```python
from build123d import *

# Parameters (mm, degrees)
SKETCH1_W           = 30
SKETCH1_H           = 9
BOSS_EXTRUDE1_DEPTH = 4
SKETCH2_W           = 34
SKETCH2_H           = 13
SKETCH2_W_2         = 30
SKETCH2_H_2         = 9
BOSS_EXTRUDE2_DEPTH = 36


with BuildPart() as part:
    # Sketch1 → Boss-Extrude1 (new body)
    with BuildSketch(Plane.XY):
        Polygon((-17, 6.5), (-17, -6.5), (-5.5, -6.5), (-5.5, -5.5), (5.5, -5.5), (5.5, -6.5), (17, -6.5), (17, 6.5), align=None)
        Rectangle(SKETCH1_W, SKETCH1_H, mode=Mode.SUBTRACT)
    extrude(amount=BOSS_EXTRUDE1_DEPTH)

    # Sketch2 → Boss-Extrude2 (add)
    with BuildSketch(Plane.XY.offset(4)):
        Rectangle(SKETCH2_W, SKETCH2_H)
        Rectangle(SKETCH2_W_2, SKETCH2_H_2, mode=Mode.SUBTRACT)
    extrude(amount=BOSS_EXTRUDE2_DEPTH)


solid = part.part
```
Model file for the job. Use its own axes, mm. A direction names the side the tool comes from. Give positions to 0.01 mm unless a question says otherwise; leave off trailing zeros. Write each loop counter-clockwise with the first axis right and the second up, starting at its lowest first coordinate (ties: lowest second). Pieces come first, ordered by that corner, then holes. Notation, with made-up numbers: (-11, 76.5) -> (17, 76.5) arc R18 cw to (17, 98.5) -> close; hole circle Ø11 at (28, 8.25). An arc over 180 degrees is marked (long way). Use CSV: the item, a comma, the result in double quotes. Start each with the question number.
1) Cut at A-A on x = -10. List the corners of the cut face in (y, z), plus the area to 3 significant figures.
2) Pin check, flat tips, straight feed: P1, Ø2, axis at x = -11, y = -2, coming from the +Z side; P2, Ø0.8, axis at x = -1.5, y = -6, coming from the -Z side; P3, Ø2, axis at x = 2.5, z = 2, coming from the -Y side. Stop position of each tip, or through.
3) Drill centre lines: L1, parallel to Y at x = 1.5, z = 16; L2, parallel to X at y = -1, z = 24. Where is each one in solid material? Low to high.
4) Two-plate mould, pull along Y, no slides. Class faces 1 (the flat face through (0, 6.5, 20)), 2 (the flat face through (0, -5.5, 2)), 3 (the flat face through (5.5, -6, 2)), 4 (the flat face through (0, 4.5, 20)): released by +Y, released by -Y, zero draft, split by the parting line, or undercut.
5) Tool access for faces 5 (the flat face through (0, -4.5, 20)), 6 (the flat face through (17, 0, 20)), 7 (the flat face through (-5.5, -6, 2)): list every direction of +Z, -Z, +X, -X, +Y, -Y with a clear straight run to the whole face (end or side of a thin tool).
6) Cut at B-B on z = 31. List the corners of the cut face in (x, y), plus the area to 3 significant figures.
7) Cut at C-C on y = -2.25. List the corners of the cut face in (x, z).
8) Cut at D-D on x = -2. List the corners of the cut face in (y, z), plus the area to 3 significant figures.
Final values:
1,outline,"(-6.5, 0) -> (-4.5, 0) -> (-4.5, 40) -> (-6.5, 40) -> close; (4.5, 0) -> (6.5, 0) -> (6.5, 40) -> (4.5, 40) -> close"
1,area,"160 mm2"
2,P1,"passes through"
2,P2,"stops at z = 4"
2,P3,"stops at y = -5.5"
3,L1,"y = -6.5 to -4.5, 4.5 to 6.5"
3,L2,"x = -17 to -15, 15 to 17"
4,face 1,"released by +Y"
4,face 2,"released by -Y"
4,face 3,"zero draft"
4,face 4,"undercut"
5,face 5,"+Z, -Z"
5,face 6,"+Z, -Z, +X, +Y, -Y"
5,face 7,"-Z, -Y"
6,outline,"(-17, -6.5) -> (17, -6.5) -> (17, 6.5) -> (-17, 6.5) -> close; hole (-15, -4.5) -> (15, -4.5) -> (15, 4.5) -> (-15, 4.5) -> close"
6,area,"172 mm2"
7,outline,"(-17, 0) -> (-15, 0) -> (-15, 40) -> (-17, 40) -> close; (15, 0) -> (17, 0) -> (17, 40) -> (15, 40) -> close"
8,outline,"(-6.5, 4) -> (-5.5, 4) -> (-5.5, 0) -> (-4.5, 0) -> (-4.5, 40) -> (-6.5, 40) -> close; (4.5, 0) -> (6.5, 0) -> (6.5, 40) -> (4.5, 40) -> close"
8,area,"156 mm2"
